Read the model definition and answer for the solid it produces. Units are mm, in the model's axes. A direction names the side the tool comes from. Coordinates: 2 decimals unless noted, no trailing zeros. Write each loop counter-clockwise with the first axis right and the second up, starting at its lowest first coordinate (ties: lowest second). Pieces come first, ordered by that corner, then holes.
1) Which of the six approach directions +Z, -Z, +X, -X, +Y, -Y give full straight-line access (tool end or side, diameter ignored) to faces 1 (the face through (-22.37, 0.95, 12.88)), 2 (the face through (7, 15, 25.4))?
2) Each of these flat-tipped pins is pushed along its axis until it touches: pin 1 Ø10 at (y, z) = (-13, 11) entering from +X; pin 2 Ø8.5 at (x, y) = (0, -25.4) entering from +Z; pin 3 Ø1 at (x, y) = (8.5, -12) entering from -Z; pin 4 Ø4 at (y, z) = (16.5, 13.5) entering from -X. Where does it stop, or does it pass through?
3) The part is cut by section A-A (y = -25.4). Determine the outline of the cut face in (x, z) (3 decimals), then the cut area to 3 significant figures.
4) Determine the mould class of faces 3 (the face through (-3.441, -15.497, 31.661)), 4 (the face through (-0.41, 28.55, 12.88)), 5 (the face through (7, 8, 0)) for opening direction X: +X half, -X half, draft (parallel to the pull), parting line (faces both ways), or undercut.
5) The part is cut by section B-B (x = 0). Determine the outline of the cut face in (y, z) (3 decimals).
6) Find the intervals of material crossed by line 1 (Y direction, x = 0, z = 8) (3 decimals); line 2 (Y direction, x = -1.5, z = 14); line 3 (Z direction, x = 16.5, y = 20), in increasing order.
7) The part is cut by section C-C (z = 4). Determine the outline of the cut face in (x, y) (3 decimals).
from build123d import *

# Parameters (mm, degrees)
F0_R     = 31.75
F1_DEPTH = 25.4
F2_R     = 15.875
F3_DEPTH = 12.7
F4_R     = 9.525
F5_DEPTH = 38.101
F6_R     = 3.175
F7_DEPTH = 25.401


with BuildPart() as f1:
    # F0 (on Top) → F1 (new body)
    with BuildSketch(Plane.XY):
        Circle(F0_R)
    extrude(amount=F1_DEPTH)

    # F2 (on face) → F3 (join)
    with BuildSketch(Plane.XY.offset(25.4)):
        Circle(F2_R)
    extrude(amount=F3_DEPTH)

    # F4 (on face) → F5 (cut, through all)
    with BuildSketch(Plane.XY.offset(38.1)):
        Circle(F4_R)
    extrude(amount=-F5_DEPTH, mode=Mode.SUBTRACT)

    # F6 (on face) → F7 (cut, through all)
    with BuildSketch(Plane.XY.offset(25.4)):
        with Locations((0, 25.4)):
            Circle(F6_R)
        with Locations((-25.4, 0)):
            Circle(F6_R)
        with Locations((0, -25.4)):
            Circle(F6_R)
        with Locations((25.4, 0)):
            Circle(F6_R)
    extrude(amount=-F7_DEPTH, mode=Mode.SUBTRACT)


solid = f1.part
Reported:
1. face 1: +Z, -Z
1. face 2: +Z
2. pin 1: stops at x = 30.73
2. pin 2: stops at z = 25.4
2. pin 3: stops at z = 0
2. pin 4: stops at x = -28.25
3. outline: (-19.05, 0) - (-3.175, 0) - (-3.175, 25.4) - (-19.05, 25.4) - close; (3.175, 0) - (19.05, 0) - (19.05, 25.4) - (3.175, 25.4) - close
3. area: 806 mm2
4. face 3: parting line
4. face 4: undercut
4. face 5: draft
5. outline: (-31.75, 0) - (-28.575, 0) - (-28.575, 25.4) - (-31.75, 25.4) - close; (-22.225, 0) - (-9.525, 0) - (-9.525, 38.1) - (-15.875, 38.1) - (-15.875, 25.4) - (-22.225, 25.4) - close; (9.525, 0) - (22.225, 0) - (22.225, 25.4) - (15.875, 25.4) - (15.875, 38.1) - (9.525, 38.1) - close; (28.575, 0) - (31.75, 0) - (31.75, 25.4) - (28.575, 25.4) - close
6. line 1: y = -31.75 to -28.575, -22.225 to -9.525, 9.525 to 22.225, 28.575 to 31.75
6. line 2: y = -31.71 to -28.2, -22.6 to -9.41, 9.41 to 22.6, 28.2 to 31.71
6. line 3: z = 0 to 25.4
7. outline: circle Ø63.5 at (0, 0); hole circle Ø6.35 at (-25.4, 0); hole circle Ø19.05 at (0, 0); hole circle Ø6.35 at (0, -25.4); hole circle Ø6.35 at (0, 25.4); hole circle Ø6.35 at (25.4, 0)
